Geometry check sheet. Reference: the model listing, model coordinates, mm. Give positions to 0.01 mm unless a question says otherwise; leave off trailing zeros. Write item = value, one per line. Start each with the question number.
(1) Section check A-A, the plane y = -1. Give the number of separate pieces and of enclosed holes in the cut face, plus the area to 3 significant figures.
(2) Depth check by flat-ended pin: pin 1 Ø3 at (x, z) = (25, -225) entering from +Y. Enter the tip coordinate at first touch or a pass-through.
(3) Thickness scan on L1, parallel to X at y = -2.6, z = -25; L2, parallel to Z at x = 25, y = -3.65; L3, parallel to Z at x = 26.5, y = -1.6. Record the ranges inside material, lowest first.
```python
from build123d import *

# Parameters (mm, degrees)
F0_W     = 250
F0_H     = 250
F1_DEPTH = 5
F2_D     = 4.8


with BuildPart() as f1:
    # F0 (on Front) → F1 (new body)
    with BuildSketch(Plane.XZ):
        with Locations((125, -125)):
            Rectangle(F0_W, F0_H)
        with BuildLine():
            ThreePointArc((41.0619131156, -149.2449066583), (36.0619131156, -154.2449066583), (31.0619131156, -149.2449066583))
            Line((31.0619131156, -149.2449066583), (34.7619131156, -137.8727704287))
            Line((34.7619131156, -137.8727704287), (35.1619131156, -99.2449066583))
            ThreePointArc((35.1619131156, -99.2449066583), (36.0619131156, -98.3449066583), (36.9619131156, -99.2449066583))
            Line((36.9619131156, -99.2449066583), (37.3619131156, -137.8727704287))
            Line((37.3619131156, -137.8727704287), (41.0619131156, -149.2449066583))
        make_face(mode=Mode.SUBTRACT)
        with BuildLine():
            Line((62.3619131156, -137.8727704287), (66.0619131156, -149.2449066583))
            ThreePointArc((66.0619131156, -149.2449066583), (61.0619131156, -154.2449066583), (56.0619131156, -149.2449066583))
            Line((56.0619131156, -149.2449066583), (59.7619131156, -137.8727704287))
            Line((59.7619131156, -137.8727704287), (60.1619131156, -99.2449066583))
            ThreePointArc((60.1619131156, -99.2449066583), (61.0619131156, -98.3449066583), (61.9619131156, -99.2449066583))
            Line((61.9619131156, -99.2449066583), (62.3619131156, -137.8727704287))
        make_face(mode=Mode.SUBTRACT)
        with BuildLine():
            Line((87.3619131156, -137.8727704287), (91.0619131156, -149.2449066583))
            ThreePointArc((91.0619131156, -149.2449066583), (86.0619131156, -154.2449066583), (81.0619131156, -149.2449066583))
            Line((81.0619131156, -149.2449066583), (84.7619131156, -137.8727704287))
            Line((84.7619131156, -137.8727704287), (85.1619131156, -99.2449066583))
            ThreePointArc((85.1619131156, -99.2449066583), (86.0619131156, -98.3449066583), (86.9619131156, -99.2449066583))
            Line((86.9619131156, -99.2449066583), (87.3619131156, -137.8727704287))
        make_face(mode=Mode.SUBTRACT)
        with BuildLine():
            Line((112.3619131156, -137.8727704287), (116.0619131156, -149.2449066583))
            ThreePointArc((116.0619131156, -149.2449066583), (111.0619131156, -154.2449066583), (106.0619131156, -149.2449066583))
            Line((106.0619131156, -149.2449066583), (109.7619131156, -137.8727704287))
            Line((109.7619131156, -137.8727704287), (110.1619131156, -99.2449066583))
            ThreePointArc((110.1619131156, -99.2449066583), (111.0619131156, -98.3449066583), (111.9619131156, -99.2449066583))
            Line((111.9619131156, -99.2449066583), (112.3619131156, -137.8727704287))
        make_face(mode=Mode.SUBTRACT)
        with BuildLine():
            Line((137.3619131156, -137.8727704287), (141.0619131156, -149.2449066583))
            ThreePointArc((141.0619131156, -149.2449066583), (136.0619131156, -154.2449066583), (131.0619131156, -149.2449066583))
            Line((131.0619131156, -149.2449066583), (134.7619131156, -137.8727704287))
            Line((134.7619131156, -137.8727704287), (135.1619131156, -99.2449066583))
            ThreePointArc((135.1619131156, -99.2449066583), (136.0619131156, -98.3449066583), (136.9619131156, -99.2449066583))
            Line((136.9619131156, -99.2449066583), (137.3619131156, -137.8727704287))
        make_face(mode=Mode.SUBTRACT)
        with BuildLine():
            Line((162.3619131156, -137.8727704287), (166.0619131156, -149.2449066583))
            ThreePointArc((166.0619131156, -149.2449066583), (161.0619131156, -154.2449066583), (156.0619131156, -149.2449066583))
            Line((156.0619131156, -149.2449066583), (159.7619131156, -137.8727704287))
            Line((159.7619131156, -137.8727704287), (160.1619131156, -99.2449066583))
            ThreePointArc((160.1619131156, -99.2449066583), (161.0619131156, -98.3449066583), (161.9619131156, -99.2449066583))
            Line((161.9619131156, -99.2449066583), (162.3619131156, -137.8727704287))
        make_face(mode=Mode.SUBTRACT)
        with BuildLine():
            Line((187.3619131156, -137.8727704287), (191.0619131156, -149.2449066583))
            ThreePointArc((191.0619131156, -149.2449066583), (186.0619131156, -154.2449066583), (181.0619131156, -149.2449066583))
            Line((181.0619131156, -149.2449066583), (184.7619131156, -137.8727704287))
            Line((184.7619131156, -137.8727704287), (185.1619131156, -99.2449066583))
            ThreePointArc((185.1619131156, -99.2449066583), (186.0619131156, -98.3449066583), (186.9619131156, -99.2449066583))
            Line((186.9619131156, -99.2449066583), (187.3619131156, -137.8727704287))
        make_face(mode=Mode.SUBTRACT)
        with BuildLine():
            Line((212.3619131156, -137.8727704287), (216.0619131156, -149.2449066583))
            ThreePointArc((216.0619131156, -149.2449066583), (211.0619131156, -154.2449066583), (206.0619131156, -149.2449066583))
            Line((206.0619131156, -149.2449066583), (209.7619131156, -137.8727704287))
            Line((209.7619131156, -137.8727704287), (210.1619131156, -99.2449066583))
            ThreePointArc((210.1619131156, -99.2449066583), (211.0619131156, -98.3449066583), (211.9619131156, -99.2449066583))
            Line((211.9619131156, -99.2449066583), (212.3619131156, -137.8727704287))
        make_face(mode=Mode.SUBTRACT)
    extrude(amount=F1_DEPTH)

    # F2 (through all)
    with Locations(Plane(origin=(0, 0, 0), x_dir=(1, 0, 0), z_dir=(0, 1, 0))):
        with Locations((25, 25), (225, 25), (225, 225), (25, 225)):
            Hole(F2_D / 2)


solid = f1.part
```
Model answer:
q1.separate_pieces = 1
q1.enclosed_holes = 12
q1.area = 60,900 mm²
q2.pin_1 = through
q3.L1 = 0 to 22.6, 27.4 to 222.6, 227.4 to 250
q3.L2 = -250 to -227.4, -222.6 to -27.4, -22.6 to 0
q3.L3 = -250 to -226.87, -223.13 to -26.87, -23.13 to 0
